Read the model definition and answer for the solid it produces. Units are mm, in the model's axes. A direction names the side the tool comes from. Give positions to 0.01 mm unless a question says otherwise; leave off trailing zeros. Write each loop counter-clockwise with the first axis right and the second up, starting at its lowest first coordinate (ties: lowest second). Pieces come first, ordered by that corner, then holes. Notation, with made-up numbers: (48.25, 33) -> (67.25, 33) arc R14 cw to (67.25, 50) -> close; hole circle Ø7 at (8, 53). An arc over 180 degrees is marked (long way). Use a Markdown table: item, result.
Autodesk Inventor part; units mm, degrees
ref_plane "РабПлоскость1" through (0, 0, 80) normal (0, 0, 1) x (1, 0, 0)
ref_plane "YZ Plane" through (0, 0, 0) normal (1, 0, 0) x (0, 1, 0)
ref_plane "XZ Plane" through (0, 0, 0) normal (0, 1, 0) x (-1, 0, 0)
sketch "Эскиз1" plane through (0, 0, 0) normal (0, 0, 1) x (1, 0, 0)
  line L0 (-43.3013, 0) -> (21.6506, 37.5)
  line L1 (21.6506, 37.5) -> (21.6506, -37.5)
  line L2 (21.6506, -37.5) -> (-43.3013, 0)
  point P0 (0, 0)
  point P1 (0, 0)
  dimension "d2" = 75
ref_plane "РабПлоскость1" through (0, 0, 80) normal (0, 0, 1) x (1, 0, 0)
sketch "Эскиз2" plane through (0, 0, 80) normal (0, 0, 1) x (1, 0, 0)
  point P0 (0, 0)
  point P1 (0, 0)
loft "Лофт1" add profiles "Эскиз1" section 2 point at (0, 0, 80)
sketch "Эскиз3" plane through (0, 0, 0) normal (0, 1, 0) x (-1, 0, 0)
  point P0 (0, 0)
sketch "Эскиз4" plane through (0, 0, 0) normal (0, 1, 0) x (-1, 0, 0)
  line L0 (-5, 10) -> (15, 10)
  line L1 (15, 10) -> (15, 40)
  line L2 (15, 40) -> (-5, 40)
  line L3 (-5, 40) -> (-5, 10)
  line L4 (-5, 10) -> (15, 40) construction
  line L5 (15, 10) -> (-5, 40) construction
  point P0 (0, 0)
  point P1 (0, 0)
  point P2 (5, 25)
  dimension "d8" = 20
  dimension "d9" = 30
  dimension "d10" = 15
  dimension "d12" = 10
extrude "Выдавливание1" cut sketch "Эскиз4" along normal through all both and the other way through all
sketch "Эскиз5" plane through (21.6506, -37.5, 0) normal (-0.4826376, -0.8359528, 0.2612353) x (0.8428609, -0.3622752, 0.3979224)
  point P0 (-31.8338, 20.6119)
properties part number "ДЗ2 Курганова"
Item 1: Each of these flat-tipped pins is pushed along its axis until it touches: P1, Ø6, axis at x = -1.5, y = 6, coming from the -Z side; P2, Ø8, axis at y = -18.5, z = 34.5, coming from the +X side; P3, Ø4, axis at x = -14.5, z = 10.5, coming from the -Y side; P4, Ø8, axis at y = 5.5, z = 27.5, coming from the +X side. Where does it stop, or does it pass through?
Return value:
| item | result |
|---|---|
| P1 | z = 0 |
| P2 | x = 13.4 |
| P3 | y = -14.66 |
| P4 | x = 15.29 |
Item 2: A cutting plane is placed at A-A (z = 16.5). Give the vertices of the cut face in (x, y).
Return value:
| item | result |
|---|---|
| outline | (-34.37, 0) -> (-15, -11.18) -> (-15, 11.18) -> close; (5, -22.73) -> (17.19, -29.77) -> (17.19, 29.77) -> (5, 22.73) -> close |
Item 3: A cutting plane is placed at D-D (x = -34). Give the vertices of the cut face in (y, z).
Return value:
| item | result |
|---|---|
| outline | (-5.37, 0) -> (5.37, 0) -> (0, 17.18) -> close |
Item 4: For a pull along X with two mould halves and no side action, classify faces 3 (the face through (13.08, -0.52, 31.67)), 4 (the face through (-3, 0, 40)), 5 (the face through (5, 0, 25)), 6 (the face through (-15.414, -8.981, 22.782)) as +X half, -X half, draft (parallel to the pull), parting line (faces both ways), or undercut.
Return value:
| item | result |
|---|---|
| face 3 | +X half |
| face 4 | undercut |
| face 5 | undercut |
| face 6 | -X half |
Item 5: A tool of negligible diameter and unlimited length cuts with its end or side. For faces 1 (the face through (2, -4, 0)), 2 (the face through (-15, 0, 21)), from which of +Z, -Z, +X, -X, +Y, -Y can it reach the whole face along a straight path? Write none if from no direction.
Return value:
| item | result |
|---|---|
| face 1 | -Z, +X, -X, +Y, -Y |
| face 2 | +Y, -Y |
Item 6: A cutting plane is placed at B-B (y = 2). Give the vertices of the cut face in (x, z), then the cut area to 3 significant figures.
Return value:
| item | result |
|---|---|
| outline | (-39.84, 0) -> (21.65, 0) -> (1.15, 75.73) -> close; hole (-15, 10) -> (5, 10) -> (5, 40) -> (-15, 40) -> close |
| area | 1,730 mm^2 |
Item 7: Straight lines are drawn through the part: line 1 along Z through (x, y) = (-3, 11); line 2 along Y through (x, z) = (5.5, 4); line 3 along X through (y, z) = (3, 39). For each, find the intervals that lie inside material, in ascending order. Write a range as [from, to].
Return value:
| item | result |
|---|---|
| line 1 | [0, 10] |
| line 2 | [-26.93, 26.93] |
| line 3 | [-17, -15], [5, 11.1] |
Item 8: A cutting plane is placed at C-C (x = -11.5). Give the vertices of the cut face in (y, z).
Return value:
| item | result |
|---|---|
| outline | (-18.36, 0) -> (18.36, 0) -> (15.24, 10) -> (-15.24, 10) -> close; (-5.86, 40) -> (5.86, 40) -> (0, 58.75) -> close |
